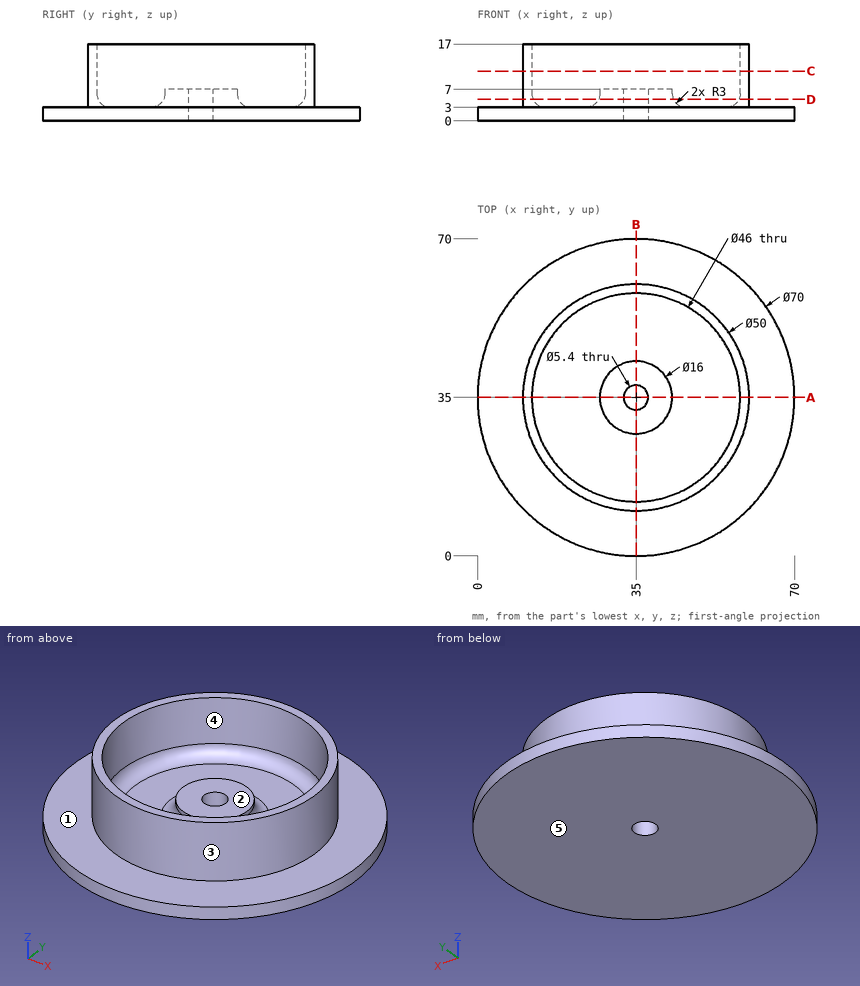
Input: dimensioned drawing with shaded views. Units: mm. Origin: part minimum x, y, z. A direction names the side the tool comes from. Give positions to 0.01 mm unless a question says otherwise; leave off trailing zeros. Write each loop counter-clockwise with the first axis right and the second up, starting at its lowest first coordinate (ties: lowest second). Pieces come first, ordered by that corner, then holes. Notation, with made-up numbers: M 52,53.25 L 96,53.25 A23 ccw 96,62.25 Z; hole C 22,3.5 d8. An arc over 180 degrees is marked long. Return JSON: item names as keys, results as strings. Group by question number.
1) Cut plane D-D, the plane z = 4.75. Output: boundary loops of the cut face in (x, y).
2) Cut plane A-A, the plane y = 35. Output: boundary loops of the cut face in (x, z).
3) Cut plane C-C, the plane z = 11. Output: boundary loops of the cut face in (x, y), plus the area to 3 significant figures.
4) Pull-direction query (Y, two-part tool) for the marked faces 1, 2 and 3; classes: pulls with the +Y half, pulls with the -Y half, needs draft (parallel to the pull), parting line crosses it, or undercut.
5) Pin query (flat end, axial travel): P1, Ø10, axis at x = 23.5, z = 4.5, coming from the -Y side; P2, Ø1.5, axis at x = 56, y = 50, coming from the +Z side; P3, Ø21, axis at x = 30, y = 33, coming from the +Z side. Return the tip coordinate at first contact, or that it passes through.
6) Set-up query: the marked faces 4 and 5. Return all of +Z, -Z, +X, -X, +Y, -Y with unobstructed straight access to the full face (end or side cutting, diameter ignored); none if empty.
7) Material intervals for line 1 along Y through (x, z) = (35, 5.75); line 2 along X through (y, z) = (40, 4.25); line 3 along Y through (x, z) = (35, 14), sorted ascending. Write a range as [from, to].
Recorded:
{
 "1": {"outline": "C 35,35 d50; C 35,35 d16.55; hole C 35,35 d45.45; hole C 35,35 d5.4"},
 "2": {"outline": "M 0,0 L 32.3,0 L 32.3,7 L 27,7 L 27,6 A3 cw 24,3 L 15,3 A3 cw 12,6 L 12,17 L 10,17 L 10,3 L 0,3 Z; M 37.7,0 L 70,0 L 70,3 L 60,3 L 60,17 L 58,17 L 58,6 A3 cw 55,3 L 46,3 A3 cw 43,6 L 43,7 L 37.7,7 Z"},
 "3": {"outline": "C 35,35 d50; hole C 35,35 d46", "area": "302 mm²"},
 "4": {"face 1": "needs draft", "face 2": "undercut", "face 3": "parting line crosses it"},
 "5": {"P1": "stops at y = 0.65", "P2": "stops at z = 3", "P3": "stops at z = 7"},
 "6": {"face 4": "+Z", "face 5": "-Z, +X, -X, +Y, -Y"},
 "7": {"line 1": "y = [10, 12.01], [26.99, 32.3], [37.7, 43.01], [57.99, 60]", "line 2": "x = [10.51, 13.13], [28.05, 41.95], [56.87, 59.49]", "line 3": "y = [10, 12], [58, 60]"}
}
